Work out the finished part from the listing and answer in its coordinate system (mm). Coordinates: 2 decimals unless noted, no trailing zeros. Order: outer loops, then holes, each group sorted by start corner. A loop starts at its lowest first (then second) coordinate and runs counter-clockwise, first axis right, second up. Notation, with made-up numbers: (40, 7.25) -> (70, 7.25) arc R33 cw to (70, 37.25) -> close; hole circle Ø3 at (50.5, 17.5). An arc over 180 degrees is marked (long way). Write item = value, one per line. Start each with the question number.
Q1. Straight lines are drawn through the part: L1, parallel to Y at x = -4, z = 0.4; L2, parallel to X at y = 29, z = 1.1; L3, parallel to X at y = 67.5, z = 1.8. For each, find the intervals that lie inside material, in ascending order. Write a range as from..to.
Q2. The part is cut by section A-A, the plane y = 51. Determine the outline of the cut face in (x, z).
Q3. For a pull along X with two mould halves and no side action, classify faces 1 (the cylindrical face through (-33.02, -71.854, 0.986)), 2 (the flat face through (-3.44, -5.84, 0.99)), 3 (the cylindrical face through (4.599, 30.924, 0.986)), 4 (the cylindrical face through (7.61, -71.95, 0.99)) as +X half, -X half, draft (parallel to the pull), parting line (faces both ways), or undercut.
Q4. Flat-ended cylindrical pins translate along their axes: pin 1 (1 mm diameter, centred on y = -40.5, z = 0.5, fed in from +X); pin 2 (3 mm diameter, centred on x = -25, y = -52.5, fed in from -Z). Find the tip coordinate at first contact, or state that the pin passes through.
Q5. The part is cut by section B-B, the plane z = 0.55. Count the separate pieces of the cut face and the enclosed holes in it, plus the area to 3 significant figures.
Q6. The part is cut by section C-C, the plane y = -51. Determine the outline of the cut face in (x, z).
```python
from build123d import *

# Parameters (mm, degrees)
F0_R     = 1.5875
F0_W     = 1.5125
F0_H     = 9.125
F0_R_2   = 1.875
F1_DEPTH = 2


with BuildPart() as f1:
    # F0 (on Top) → F1 (new body)
    with BuildSketch(Plane.XY):
        with BuildLine():
            Line((-8.3077662669, 82.3469734799), (-12.6567107354, 82.3469734799))
            Line((-12.6567107354, 82.3469734799), (-17.0056552038, 82.3469734799))
            ThreePointArc((-17.0056552038, 82.3469734799), (-21.9425943503, 80.450262999), (-24.3396503152, 75.7359230148))
            ThreePointArc((-24.3396503152, 75.7359230148), (-28.1319401622, 55.4595641269), (-35.1567107354, 36.0645959539))
            Line((-35.1567107354, 36.0645959539), (-35.1567107354, 35.3542267511))
            Line((-35.1567107354, 35.3542267511), (-34.7306092033, -67.6578189428))
            ThreePointArc((-34.7306092033, -67.6578189428), (-32.9732498904, -71.9004596299), (-28.7306092033, -73.6578189428))
            Line((-28.7306092033, -73.6578189428), (3.4171877326, -73.6578189428))
            ThreePointArc((3.4171877326, -73.6578189428), (7.6598284197, -71.9004596299), (9.4171877326, -67.6578189428))
            Line((9.4171877326, -67.6578189428), (9.7246083807, 2.1247686199))
            Line((9.7246083807, 2.1247686199), (9.8432892646, 29.0645959539))
            Line((9.8432892646, 29.0645959539), (9.8432892646, 35.3542267511))
            Line((9.8432892646, 35.3542267511), (9.8432892646, 36.0645959539))
            ThreePointArc((9.8432892646, 36.0645959539), (2.8185186915, 55.4595641269), (-0.9737711555, 75.7359230148))
            ThreePointArc((-0.9737711555, 75.7359230148), (-3.3708271204, 80.450262999), (-8.3077662669, 82.3469734799))
        make_face()
        with Locations((-28.7306092033, -67.6578189428)):
            Circle(F0_R, mode=Mode.SUBTRACT)
        with Locations((-27.1615939174, -58.4994030434)):
            Rectangle(F0_W, F0_H, mode=Mode.SUBTRACT)
        with Locations((-27.1615939174, -41.3744030434)):
            Rectangle(F0_W, F0_H, mode=Mode.SUBTRACT)
        with Locations((-30.1567107354, -23.6662209918)):
            Circle(F0_R_2, mode=Mode.SUBTRACT)
        Polygon((-22.7049022828, -3.962064999), (-17.7049022828, -3.962064999), (-20.2049022828, -8.2921920179), align=None, mode=Mode.SUBTRACT)
        Polygon((-23.5629521225, 3.4575584355), (-18.5629521225, 3.4575584355), (-21.0629521225, -0.8725685834), align=None, mode=Mode.SUBTRACT)
        Polygon((-15.23480489, -7.3942718085), (-10.23480489, -7.3942718085), (-12.73480489, -11.7243988275), align=None, mode=Mode.SUBTRACT)
        with Locations((3.4171877326, -67.6578189428)):
            Circle(F0_R, mode=Mode.SUBTRACT)
        with Locations((1.3634060826, -58.4994030434)):
            Rectangle(F0_W, F0_H, mode=Mode.SUBTRACT)
        with Locations((1.3634060826, -41.3744030434)):
            Rectangle(F0_W, F0_H, mode=Mode.SUBTRACT)
        Polygon((-14.9319611404, 0.4291358414), (-9.9319611404, 0.4291358414), (-12.4319611404, -3.9009911775), align=None, mode=Mode.SUBTRACT)
        Polygon((-7.2094976817, -3.709698933), (-2.2094976817, -3.709698933), (-4.7094976817, -8.039825952), align=None, mode=Mode.SUBTRACT)
        Polygon((-7.0580758069, 3.4575584355), (-2.0580758069, 3.4575584355), (-4.5580758069, -0.8725685834), align=None, mode=Mode.SUBTRACT)
        with Locations((4.8432892646, -23.6662209918)):
            Circle(F0_R_2, mode=Mode.SUBTRACT)
        with Locations((-30.1567107354, 29.0645959539)):
            Circle(F0_R_2, mode=Mode.SUBTRACT)
        Polygon((-23.1448143635, 10.267657322), (-18.1448143635, 10.267657322), (-20.6448143635, 5.9375303031), align=None, mode=Mode.SUBTRACT)
        Polygon((-15.2871601198, 15.2332606736), (-10.2871601198, 15.2332606736), (-12.7871601198, 10.9031336547), align=None, mode=Mode.SUBTRACT)
        Polygon((-19.9925371002, 59.3395778543), (-14.9925371002, 59.3395778543), (-17.4925371002, 55.0094508354), align=None, mode=Mode.SUBTRACT)
        Polygon((-15.2093276296, 56.7469392914), (-10.2093276296, 56.7469392914), (-12.7093276296, 52.4168122725), align=None, mode=Mode.SUBTRACT)
        Polygon((-15.3613381002, 62.3649583209), (-10.3613381002, 62.3649583209), (-12.8613381002, 58.034831302), align=None, mode=Mode.SUBTRACT)
        Polygon((-20.0741064349, 65.0715577427), (-15.0741064349, 65.0715577427), (-17.5741064349, 60.7414307238), align=None, mode=Mode.SUBTRACT)
        Polygon((-19.9925371002, 70.1445944501), (-14.9925371002, 70.1445944501), (-17.4925371002, 65.8144674312), align=None, mode=Mode.SUBTRACT)
        Polygon((-15.2171917174, 72.7440145343), (-10.2171917174, 72.7440145343), (-12.7171917174, 68.4138875154), align=None, mode=Mode.SUBTRACT)
        Polygon((-14.7060893391, 7.8873719099), (-9.7060893391, 7.8873719099), (-12.2060893391, 3.557244891), align=None, mode=Mode.SUBTRACT)
        Polygon((-6.4523920331, 10.3219720546), (-1.4523920331, 10.3219720546), (-3.9523920331, 5.9918450356), align=None, mode=Mode.SUBTRACT)
        with Locations((4.8432892646, 29.0645959539)):
            Circle(F0_R_2, mode=Mode.SUBTRACT)
        Polygon((-10.6306696928, 59.3395778543), (-5.6306696928, 59.3395778543), (-8.1306696928, 55.0094508354), align=None, mode=Mode.SUBTRACT)
        Polygon((-15.1065990243, 67.459733436), (-10.1065990243, 67.459733436), (-12.6065990243, 63.1296064171), align=None, mode=Mode.SUBTRACT)
        Polygon((-10.3938269644, 65.0715577427), (-5.3938269644, 65.0715577427), (-7.8938269644, 60.7414307238), align=None, mode=Mode.SUBTRACT)
        Polygon((-10.0930306195, 70.1445944501), (-5.0930306195, 70.1445944501), (-7.5930306195, 65.8144674312), align=None, mode=Mode.SUBTRACT)
        with Locations((-12.6567107354, 77.3469734799)):
            Circle(F0_R, mode=Mode.SUBTRACT)
    extrude(amount=F1_DEPTH)


solid = f1.part
```
Model answer:
q1.L1 = -73.66..-6.81, -3.71..0.09, 3.46..6.07, 10.32..80.96
q1.L2 = -35.13..-32.03, -28.28..2.97, 6.72..9.84
q1.L3 = -25.47..-18.47, -16.52..-8.57, -6.62..0.16
q2.outline = (-29.44, 0) -> (4.12, 0) -> (4.12, 2) -> (-29.44, 2) -> close
q3.face_1 = -X half
q3.face_2 = undercut
q3.face_3 = undercut
q3.face_4 = +X half
q4.pin_1 = 9.54
q4.pin_2 = 0
q5.separate_pieces = 1
q5.enclosed_holes = 31
q5.area = 5,930 mm2
q6.outline = (-34.8, 0) -> (9.49, 0) -> (9.49, 2) -> (-34.8, 2) -> close
